Model file for the job. Use its own axes, mm. A direction names the side the tool comes from. Round coordinates to 2 decimals unless told otherwise and drop trailing zeros. Order: outer loops, then holes, each group sorted by start corner. A loop starts at its lowest first (then second) coordinate and runs counter-clockwise, first axis right, second up. Notation, with made-up numbers: (-29.5, 8) - (13.5, 8) arc R21 ccw to (13.5, 16) - close; hole circle Ø3 at (2.5, -29.75). An arc over 180 degrees is marked (long way). Answer as CSV lines item,"result". Start each with the question number.
1. Wall check: line 1 along X through (y, z) = (24.8, 11); line 2 along Z through (x, y) = (14, 24.9); line 3 along Z through (x, y) = (47, 22.7). Give the ranges that are in metal, low to high. Write a range as [from, to].
2. Band-saw the part on C-C on y = 25.5. List the corners of the cut face in (x, z), then the cut area to 3 significant figures.
3. Pin check, flat tips, straight feed: pin 1 Ø1.5 at (x, y) = (14.5, 23.5) entering from -Z; pin 2 Ø1.5 at (x, y) = (54, 23) entering from +Z. Stop position of each tip, or through.
4. Band-saw the part on B-B on x = 14. List the corners of the cut face in (y, z).
5. 3-axis set-ups, long thin cutter, end or side, ignore diameter. For faces 4 (the face through (55, 24, 10)), 5 (the face through (22.005, 23.994, 109.27)), 6 (the face through (9.47, 24, 52)): which of +Z, -Z, +X, -X, +Y, -Y reach the whole face in a straight line?
6. Band-saw the part on A-A on z = 89. List the corners of the cut face in (x, y), then the cut area to 3 significant figures.
7. Pull direction X, two halves, no side cores. Call faces 1 (the face through (34, 24, 0)), 2 (the face through (51.97, 24, 20)), 3 (the face through (47.005, 23.994, 109.391)): released by +X, released by -X, zero draft, split by the parting line, or undercut.
Autodesk Inventor part; units mm, degrees
ref_plane "YZ Plane" through (0, 0, 0) normal (1, 0, 0) x (0, 1, 0)
ref_plane "XZ Plane" through (0, 0, 0) normal (0, 1, 0) x (-1, 0, 0)
ref_plane "XY Plane" through (0, 0, 0) normal (0, 0, 1) x (1, 0, 0)
sketch "Sketch1" plane through (0, 0, 0) normal (0, 0, 1) x (1, 0, 0)
  line L0 (9.4704, 26.4594) -> (59.4704, 26.4594)
  line L1 (59.4704, 26.4594) -> (59.4704, 21.4594)
  line L2 (59.4704, 21.4594) -> (9.4704, 21.4594)
  line L3 (9.4704, 21.4594) -> (9.4704, 26.4594)
  point P0 (0, 0)
  dimension "d0" = 50
  dimension "d1" = 5
extrude "Extrusion1" add sketch "Sketch1" along normal blind 105
sketch "Sketch2" plane through (9.4704, 26.4594, 0) normal (0, 1, 0) x (1, 0, 0)
  line L0 (0, -105) -> (50, -105)
  line L1 (0, 0) -> (50, 0)
  line L2 (0, -105) -> (50, -105)
  line L3 (50, -105) -> (50, 0)
  line L4 (50, 0) -> (0, 0)
  line L5 (0, 0) -> (0, -105)
  line L6 (2.5, -95) -> (7.5, -95)
  line L7 (7.5, -95) -> (7.5, -74)
  line L8 (7.5, -74) -> (2.5, -74)
  line L9 (2.5, -74) -> (2.5, -95)
  line L10 (42.5, -95) -> (47.5, -95)
  line L11 (47.5, -95) -> (47.5, -74)
  line L12 (47.5, -74) -> (42.5, -74)
  line L13 (42.5, -74) -> (42.5, -95)
  line L14 (42.5, -31) -> (47.5, -31)
  line L15 (47.5, -31) -> (47.5, -10)
  line L16 (47.5, -10) -> (42.5, -10)
  line L17 (42.5, -10) -> (42.5, -31)
  line L18 (2.5, -31) -> (7.5, -31)
  line L19 (7.5, -31) -> (7.5, -10)
  line L20 (7.5, -10) -> (2.5, -10)
  line L21 (2.5, -10) -> (2.5, -31)
  line L22 (15, -105) -> (10, -113.6603)
  line L23 (15, -105) -> (25, -105) construction
  line L24 (10, -113.6603) -> (40, -113.6603)
  line L25 (40, -113.6603) -> (35, -105)
  point P0 (-9.4704, 0)
  dimension "d4" = 5
  dimension "d5" = 21
  dimension "d6" = 5
  dimension "d7" = 21
  dimension "d8" = 5
  dimension "d9" = 21
  dimension "d10" = 5
  dimension "d11" = 21
  dimension "d12" = 2.5
  dimension "d13" = 2.5
  dimension "d14" = 2.5
  dimension "d15" = 2.5
  dimension "d16" = 10
  dimension "d17" = 10
  dimension "d18" = 10
  dimension "d19" = 10
  dimension "d22" = 10
  dimension "d23" = 120
  dimension "d24" = 30
  dimension "d25" = 10
  dimension "d26" = 15
  dimension "d29" = 105
  dimension "d30" = 105
  dimension "d31" = 15
  dimension "d32" = 35
extrude "Extrusion2" cut sketch "Sketch2" against normal blind 105 contours L9 L8 L7 L6 | L13 L12 L11 L10 | L17 L16 L15 L14 | L21 L20 L19 L18
extrude "Extrusion3" add sketch "Sketch2" against normal blind 5 contours L0 L25 L24 L22
equation "\"d13\" = d12"
equation "\"d14\" = d12"
equation "\"d15\" = d12"
equation "\"d17\" = d16"
equation "\"d18\" = d16"
equation "\"d19\" = d16"
properties part number "inslide1"
Reply:
1,line 1,"x = [9.47, 11.97], [16.97, 51.97], [56.97, 59.47]"
1,line 2,"z = [0, 10], [31, 74], [95, 105]"
1,line 3,"z = [0, 105], [109.38, 113.66]"
2,outline,"(9.47, 0) - (59.47, 0) - (59.47, 105) - (44.47, 105) - (49.47, 113.66) - (19.47, 113.66) - (24.47, 105) - (9.47, 105) - close; hole (11.97, 10) - (16.97, 10) - (16.97, 31) - (11.97, 31) - close; hole (11.97, 74) - (16.97, 74) - (16.97, 95) - (11.97, 95) - close; hole (51.97, 10) - (56.97, 10) - (56.97, 31) - (51.97, 31) - close; hole (51.97, 74) - (56.97, 74) - (56.97, 95) - (51.97, 95) - close"
2,area,"5,050 mm2"
3,pin 1,"stops at z = 0"
3,pin 2,"stops at z = 105"
4,outline,"(21.46, 0) - (26.46, 0) - (26.46, 10) - (21.46, 10) - close; (21.46, 31) - (26.46, 31) - (26.46, 74) - (21.46, 74) - close; (21.46, 95) - (26.46, 95) - (26.46, 105) - (21.46, 105) - close"
5,face 4,"+Y, -Y"
5,face 5,"-X, +Y, -Y"
5,face 6,"+Z, -Z, -X, +Y, -Y"
6,outline,"(9.47, 21.46) - (11.97, 21.46) - (11.97, 26.46) - (9.47, 26.46) - close; (16.97, 21.46) - (51.97, 21.46) - (51.97, 26.46) - (16.97, 26.46) - close; (56.97, 21.46) - (59.47, 21.46) - (59.47, 26.46) - (56.97, 26.46) - close"
6,area,"200 mm2"
7,face 1,"zero draft"
7,face 2,"undercut"
7,face 3,"released by +X"
